The model under review builds one solid part; all positions refer to its coordinate system, in mm. Give positions to 0.01 mm unless a question says otherwise; leave off trailing zeros. Order: outer loops, then holes, each group sorted by start corner. A loop starts at its lowest first (then second) coordinate and runs counter-clockwise, first axis right, second up.
```python
from build123d import *

# Parameters (mm, degrees)
F1_DEPTH = 3.048


with BuildPart() as f1:
    # F0 (on Front) → F1 (new body)
    with BuildSketch(Plane.XZ):
        with BuildLine():
            ThreePointArc((9.4502929642, 115.490625), (0, 123.825), (-9.4502929642, 115.490625))
            ThreePointArc((-9.4502929642, 115.490625), (-7.14375, 107.9998046905), (0, 104.775))
            ThreePointArc((0, 104.775), (6.7351920908, 107.5648079092), (9.525, 114.3))
            ThreePointArc((9.525, 114.3), (9.5063048942, 114.896483242), (9.4502929642, 115.490625))
        make_face()
        with BuildLine():
            ThreePointArc((3.175, 114.3), (2.2450640303, 112.0549359697), (0, 111.125))
            ThreePointArc((0, 111.125), (-2.2450640303, 116.5450640303), (3.175, 114.3))
        make_face(mode=Mode.SUBTRACT)
        with BuildLine():
            Line((-9.4502929642, 115.490625), (-15.7504882737, 65.484375))
            ThreePointArc((-15.7504882737, 65.484375), (-10.5003255158, 75.40625), (0, 79.375))
            Line((0, 79.375), (0, 97.8521401046))
            ThreePointArc((0, 97.8521401046), (-7.0224425673, 100.0252), (0, 102.1982598954))
            Line((0, 102.1982598954), (0, 104.775))
            ThreePointArc((0, 104.775), (-7.14375, 107.9998046905), (-9.4502929642, 115.490625))
        make_face()
        with BuildLine():
            Line((0, 97.8521401046), (0, 79.375))
            ThreePointArc((0, 79.375), (10.5003255158, 75.40625), (15.7504882737, 65.484375))
            Line((15.7504882737, 65.484375), (9.4502929642, 115.490625))
            ThreePointArc((9.4502929642, 115.490625), (9.5063048942, 114.896483242), (9.525, 114.3))
            ThreePointArc((9.525, 114.3), (6.7351920908, 107.5648079092), (0, 104.775))
            Line((0, 104.775), (0, 102.1982598954))
            ThreePointArc((0, 102.1982598954), (0.5004893865, 101.1625618944), (0.6724425673, 100.0252))
            ThreePointArc((0.6724425673, 100.0252), (0.5004893865, 98.8878381056), (0, 97.8521401046))
        make_face()
        with BuildLine():
            Line((0, 47.625), (0, 7.9375))
            ThreePointArc((0, 7.9375), (5.6126600757, 5.6126600757), (7.9375, 0))
            Line((7.9375, 0), (36.5125, 0))
            ThreePointArc((36.5125, 0), (38.8373399243, 5.6126600757), (44.45, 7.9375))
            Line((44.45, 7.9375), (18.0149584735, 7.9375))
            ThreePointArc((18.0149584735, 7.9375), (12.0523084735, 10.6291369817), (10.127113946, 16.881475))
            Line((10.127113946, 16.881475), (15.7504882737, 61.515625))
            ThreePointArc((15.7504882737, 61.515625), (10.5003255158, 51.59375), (0, 47.625))
        make_face()
        with BuildLine():
            Line((0, 60.325), (0, 47.625))
            ThreePointArc((0, 47.625), (10.5003255158, 51.59375), (15.7504882737, 61.515625))
            ThreePointArc((15.7504882737, 61.515625), (15.8438414904, 62.5058612634), (15.875, 63.5))
            ThreePointArc((15.875, 63.5), (15.8438414904, 64.4941387366), (15.7504882737, 65.484375))
            ThreePointArc((15.7504882737, 65.484375), (10.5003255158, 75.40625), (0, 79.375))
            Line((0, 79.375), (0, 66.675))
            ThreePointArc((0, 66.675), (2.2450640303, 65.7450640303), (3.175, 63.5))
            ThreePointArc((3.175, 63.5), (2.2450640303, 61.2549359697), (0, 60.325))
        make_face()
        with BuildLine():
            ThreePointArc((-15.7504882737, 61.515625), (-10.5003255158, 51.59375), (0, 47.625))
            Line((0, 47.625), (0, 60.325))
            ThreePointArc((0, 60.325), (-3.175, 63.5), (0, 66.675))
            Line((0, 66.675), (0, 79.375))
            ThreePointArc((0, 79.375), (-10.5003255158, 75.40625), (-15.7504882737, 65.484375))
            ThreePointArc((-15.7504882737, 65.484375), (-15.875, 63.5), (-15.7504882737, 61.515625))
        make_face()
        with BuildLine():
            ThreePointArc((-7.8752441368, -0.9921875), (-5.953125, 5.2501627579), (0, 7.9375))
            Line((0, 7.9375), (0, 47.625))
            ThreePointArc((0, 47.625), (-10.5003255158, 51.59375), (-15.7504882737, 61.515625))
            Line((-15.7504882737, 61.515625), (-7.8752441368, -0.9921875))
        make_face()
        with BuildLine():
            Line((36.5125, 0), (7.9375, 0))
            ThreePointArc((7.9375, 0), (5.6126600757, -5.6126600757), (0, -7.9375))
            Line((0, -7.9375), (44.45, -7.9375))
            ThreePointArc((44.45, -7.9375), (38.8373399243, -5.6126600757), (36.5125, 0))
        make_face()
        with BuildLine():
            ThreePointArc((44.45, 7.9375), (38.8373399243, 5.6126600757), (36.5125, 0))
            ThreePointArc((36.5125, 0), (38.8373399243, -5.6126600757), (44.45, -7.9375))
            ThreePointArc((44.45, -7.9375), (50.0626600757, -5.6126600757), (52.3875, 0))
            ThreePointArc((52.3875, 0), (50.0626600757, 5.6126600757), (44.45, 7.9375))
        make_face()
        with BuildLine():
            ThreePointArc((47.625, 0), (44.45, -3.175), (41.275, 0))
            ThreePointArc((41.275, 0), (44.45, 3.175), (47.625, 0))
        make_face(mode=Mode.SUBTRACT)
        with BuildLine():
            ThreePointArc((3.175, 0), (-2.2450640303, -2.2450640303), (0, 3.175))
            Line((0, 3.175), (0, 7.9375))
            ThreePointArc((0, 7.9375), (-5.953125, 5.2501627579), (-7.8752441368, -0.9921875))
            ThreePointArc((-7.8752441368, -0.9921875), (-5.2501627579, -5.953125), (0, -7.9375))
            ThreePointArc((0, -7.9375), (5.6126600757, -5.6126600757), (7.9375, 0))
            Line((7.9375, 0), (3.175, 0))
        make_face()
        with BuildLine():
            Line((0, 7.9375), (0, 3.175))
            ThreePointArc((0, 3.175), (2.2450640303, 2.2450640303), (3.175, 0))
            Line((3.175, 0), (7.9375, 0))
            ThreePointArc((7.9375, 0), (5.6126600757, 5.6126600757), (0, 7.9375))
        make_face()
    extrude(amount=F1_DEPTH)


solid = f1.part
```
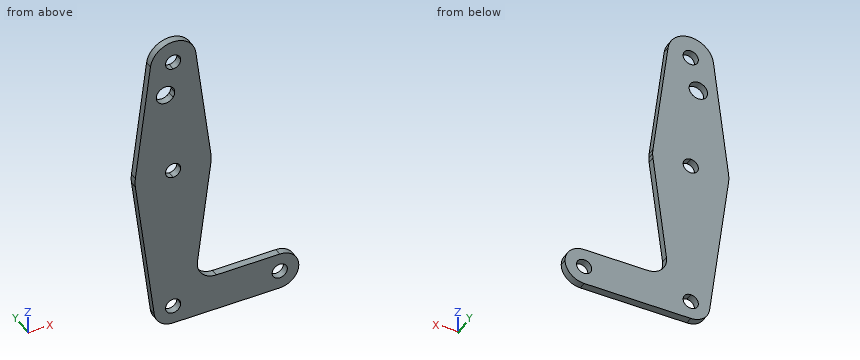
1. Take a section at A-A (y = -1.6). Count the separate pieces of the cut face and the enclosed holes in it, and give its area (3 significant figures).
2. Take a section at C-C (z = 107.5). Write out the cut boundary in (x, y), and give its area (3 significant figures).
3. To check wall thickness, follow line 1 (Z direction, x = 44.5, y = -1.25); line 2 (Z direction, x = 21.5, y = -0.3); line 3 (Z direction, x = 47, y = -1.8). State the ranges of each line that lie inside material, in increasing order.
4. Take a section at B-B (x = 31). Write out the cut boundary in (y, z), and give its area (3 significant figures).
5. Insertion check: pin 1 (1.5 mm diameter, centred on x = 30, y = -2, fed in from +Z); pin 2 (1 mm diameter, centred on y = -1, z = 34, fed in from -X); pin 3 (6 mm diameter, centred on x = -3.17, z = 100.03, fed in from +Y). Each pin has a flat end and moves straight along its axis. Give the tip position at first contact, or say it passes through.
Answer:
1. separate pieces: 1
1. enclosed holes: 5
1. area: 3,600 mm2
2. outline: (-10.46, -3.05) - (10.46, -3.05) - (10.46, 0) - (-10.46, 0) - close
2. area: 63.7 mm2
3. line 1: z = -7.94 to -3.17, 3.17 to 7.94
3. line 2: z = -7.94 to 7.94
3. line 3: z = -7.52 to -1.89, 1.89 to 7.52
4. outline: (-3.05, -7.94) - (0, -7.94) - (0, 7.94) - (-3.05, 7.94) - close
4. area: 48.4 mm2
5. pin 1: stops at z = 7.94
5. pin 2: stops at x = -12.35
5. pin 3: passes through
